```python
from build123d import *

# Parameters (mm, degrees)
SKETCH1_R           = 6.35
BOSS_EXTRUDE1_DEPTH = 104.775
SKETCH2_R           = 3.175
BOSS_EXTRUDE2_DEPTH = 12.7
FILLET1_R           = 0.508
CHAMFER1_SIZE       = 0.508


with BuildPart() as part:
    # Sketch1 → Boss-Extrude1 (new body, symmetric)
    with BuildSketch(Plane(origin=(0, 0, 0), x_dir=(1, 0, 0), z_dir=(0, 1, 0))):
        Circle(SKETCH1_R)
    extrude(amount=BOSS_EXTRUDE1_DEPTH, both=True)

    # Sketch2 → Boss-Extrude2 (add)
    with BuildSketch(Plane(origin=(0, 104.775, 0), x_dir=(1, 0, 0), z_dir=(0, 1, 0))):
        Circle(SKETCH2_R)
    extrude(amount=BOSS_EXTRUDE2_DEPTH)

    # Fillet1
    fillet1_edges = [part.edges().sort_by_distance(p)[0] for p in [
        (-3.175, 104.775, 0),
    ]]
    fillet(fillet1_edges, radius=FILLET1_R)

    # Chamfer1
    chamfer1_edges = [part.edges().sort_by_distance(p)[0] for p in [
        (-3.175, 117.475, 0),
    ]]
    chamfer(chamfer1_edges, length=CHAMFER1_SIZE)


solid = part.part
```
The listing builds one solid part. Answer for the finished solid, in the listing's coordinates (mm). A direction names the side the tool comes from. Give positions to 0.01 mm unless a question says otherwise; leave off trailing zeros. Order: outer loops, then holes, each group sorted by start corner. A loop starts at its lowest first (then second) coordinate and runs counter-clockwise, first axis right, second up. Notation, with made-up numbers: (-27, -7.5) -> (31, -7.5) arc R23 cw to (31, 0.5) -> close; hole circle Ø11 at (32, 53.5). An arc over 180 degrees is marked (long way). Answer as CSV lines item,"result". Start each with the question number.
Q1. A cutting plane is placed at B-B (x = 0). Determine the outline of the cut face in (y, z) (3 decimals), then the cut area to 3 significant figures.
Q2. A cutting plane is placed at C-C (y = -57). Determine the outline of the cut face in (x, z), then the cut area to 3 significant figures.
Q3. Find the intervals of material crossed by L1, parallel to Y at x = -5, z = -1 (3 decimals); L2, parallel to Z at x = 0.5, y = 91; L3, parallel to X at y = 2, z = -3.25, in increasing order.
Q4. Given pin 1 (2 mm diameter, centred on y = 37.5, z = -4.5, fed in from -X); pin 2 (5 mm diameter, centred on y = -42.5, z = -5, fed in from +X); pin 3 (2 mm diameter, centred on x = -4, y = 1.5, fed in from -Z), each flat-ended and moving along its own axis, determine where each tip first touches the part or whether it passes through.
Q5. A cutting plane is placed at A-A (z = 0). Determine the outline of the cut face in (x, y) (3 decimals), then the cut area to 3 significant figures.
Q6. Which of the six approach directions +Z, -Z, +X, -X, +Y, -Y give full straight-line access (tool end or side, diameter ignored) to faces 1 (the flat face through (0, 117.475, 0)), 2 (the cylindrical face through (-0.69, 111.04, 3.1))?
Results found:
1,outline,"(-104.775, -6.35) -> (104.775, -6.35) -> (104.775, -3.683) arc R0.508 cw to (105.283, -3.175) -> (116.967, -3.175) -> (117.475, -2.667) -> (117.475, 2.667) -> (116.967, 3.175) -> (105.283, 3.175) arc R0.508 cw to (104.775, 3.683) -> (104.775, 6.35) -> (-104.775, 6.35) -> close"
1,area,"2,740 mm2"
2,outline,"circle Ø12.7 at (0, 0)"
2,area,"127 mm2"
3,L1,"-104.775 to 104.775"
3,L2,"-6.33 to 6.33"
3,L3,"-5.46 to 5.46"
4,pin 1,"x = -5.3"
4,pin 2,"x = 5.84"
4,pin 3,"z = -5.6"
5,outline,"(-6.35, -104.775) -> (6.35, -104.775) -> (6.35, 104.775) -> (3.683, 104.775) arc R0.508 cw to (3.175, 105.283) -> (3.175, 116.967) -> (2.667, 117.475) -> (-2.667, 117.475) -> (-3.175, 116.967) -> (-3.175, 105.283) arc R0.508 cw to (-3.683, 104.775) -> (-6.35, 104.775) -> close"
5,area,"2,740 mm2"
6,face 1,"+Z, -Z, +X, -X, +Y"
6,face 2,"+Y"
